from build123d import *

# Parameters (mm, degrees)
BOX_W              = 10
BOX_H              = 10
BOX_DEPTH          = 10
SKETCH_W           = 4.4
SKETCH_H           = 4.4
PAD_DEPTH          = 4
PAD_FACE4_W        = 10
PAD_FACE4_H        = 10
POCKET_DEPTH       = 2.5
POCKET_FACE5_W     = 10
POCKET_FACE5_H     = 10
POCKET001_DEPTH    = 2.5
SKETCH001_W        = 5
SKETCH001_H        = 10
PAD001_DEPTH       = 10
SKETCH002_W        = 4.4
SKETCH002_H        = 4.4
PAD002_DEPTH       = 4
PAD002_FACE22_W    = 4.4
PAD002_FACE22_H    = 4.4
POCKET002_DEPTH    = 5
POCKET002_FACE16_W = 5
POCKET002_FACE16_H = 10
POCKET003_DEPTH    = 7.5
POCKET003_FACE15_W = 5
POCKET003_FACE15_H = 10
POCKET004_DEPTH    = 2.5
POCKET005_DEPTH    = 9
POCKET005_FACE8_W  = 5
POCKET005_FACE8_H  = 1
PAD003_DEPTH       = 10
PAD003_FACE3_W     = 2.5
PAD003_FACE3_H     = 1
PAD004_DEPTH       = 15
PAD004_FACE7_W     = 5
PAD004_FACE7_H     = 1
PAD005_DEPTH       = 15
PAD005_FACE8_W     = 2.5
PAD005_FACE8_H     = 1
PAD006_DEPTH       = 15
PAD006_FACE23_W    = 10
PAD006_FACE23_H    = 1
PAD007_DEPTH       = 15
SKETCH003_W        = 4.4
SKETCH003_H        = 4.4
PAD008_DEPTH       = 4
PAD008_FACE15_W    = 2.5
PAD008_FACE15_H    = 1
POCKET006_DEPTH    = 2.5
POCKET006_FACE20_W = 5
POCKET006_FACE20_H = 1
POCKET007_DEPTH    = 2.5
POCKET007_FACE27_W = 2.5
POCKET007_FACE27_H = 1
POCKET008_DEPTH    = 2.5
POCKET008_FACE37_W = 10
POCKET008_FACE37_H = 1
POCKET009_DEPTH    = 2.5
POCKET009_FACE5_W  = 10
POCKET009_FACE5_H  = 1
PAD009_DEPTH       = 2.5
PAD009_FACE29_W    = 10
PAD009_FACE29_H    = 1
PAD010_DEPTH       = 2.5
POCKET010_DEPTH    = 5


with BuildPart() as part:
    # Box → Box (new body)
    with BuildSketch(Plane.XY):
        with Locations((5, 5)):
            Rectangle(BOX_W, BOX_H)
    extrude(amount=BOX_DEPTH)

    # Sketch (on Face6 of BaseFeature) → Pad (new body)
    with BuildSketch(Plane.XY.offset(10)):
        with Locations((5, 5)):
            Rectangle(SKETCH_W, SKETCH_H)
    extrude(amount=PAD_DEPTH)

    # Pad Face4 → Pocket (cut)
    with BuildSketch(Plane(origin=(5, 10, 5), x_dir=(1, 0, 0), z_dir=(0, 1, 0))):
        Rectangle(PAD_FACE4_W, PAD_FACE4_H)
    extrude(amount=-POCKET_DEPTH, mode=Mode.SUBTRACT)

    # Pocket Face5 → Pocket001 (cut)
    with BuildSketch(Plane(origin=(5, 0, 5), x_dir=(-1, 0, 0), z_dir=(0, -1, 0))):
        Rectangle(POCKET_FACE5_W, POCKET_FACE5_H)
    extrude(amount=-POCKET001_DEPTH, mode=Mode.SUBTRACT)

    # Sketch001 (on Face3 of Pocket001) → Pad001 (join)
    with BuildSketch(Plane(origin=(0, 7.5, 0), x_dir=(-1, 0, 0), z_dir=(0, 1, 0))):
        with Locations((-5, 5)):
            Rectangle(SKETCH001_W, SKETCH001_H)
    extrude(amount=PAD001_DEPTH)

    # Sketch002 (on Face6 of Pad001) → Pad002 (join)
    with BuildSketch(Plane.XY.offset(10)):
        with Locations((5, 12.5)):
            Rectangle(SKETCH002_W, SKETCH002_H)
    extrude(amount=PAD002_DEPTH)

    # Pad002 Face22 → Pocket002 (cut)
    with BuildSketch(Plane(origin=(5, 12.5, 14), x_dir=(0, 1, 0), z_dir=(0, 0, 1))):
        Rectangle(PAD002_FACE22_W, PAD002_FACE22_H)
    extrude(amount=-POCKET002_DEPTH, mode=Mode.SUBTRACT)

    # Pocket002 Face16 → Pocket003 (cut)
    with BuildSketch(Plane(origin=(5, 17.5, 5), x_dir=(1, 0, 0), z_dir=(0, 1, 0))):
        Rectangle(POCKET002_FACE16_W, POCKET002_FACE16_H)
    extrude(amount=-POCKET003_DEPTH, mode=Mode.SUBTRACT)

    # Pocket003 Face15 → Pocket004 (cut)
    with BuildSketch(Plane(origin=(5, 10, 5), x_dir=(1, 0, 0), z_dir=(0, 1, 0))):
        Rectangle(POCKET003_FACE15_W, POCKET003_FACE15_H)
    extrude(amount=-POCKET004_DEPTH, mode=Mode.SUBTRACT)

    # Pocket004 Face4 → Pocket005 (cut)
    with BuildSketch(Plane(origin=(5, 5, 0), x_dir=(0, -1, 0), z_dir=(0, 0, -1))):
        Polygon((2.5, 5), (-2.5, 5), (-2.5, 2.5), (-2.5, -2.5), (-2.5, -5), (2.5, -5), align=None)
    extrude(amount=-POCKET005_DEPTH, mode=Mode.SUBTRACT)

    # Pocket005 Face8 → Pad003 (add)
    with BuildSketch(Plane(origin=(10, 5, 9.5), x_dir=(0, -1, 0), z_dir=(1, 0, 0))):
        Rectangle(POCKET005_FACE8_W, POCKET005_FACE8_H)
    extrude(amount=PAD003_DEPTH)

    # Pad003 Face3 → Pad004 (add)
    with BuildSketch(Plane(origin=(1.25, 7.5, 9.5), x_dir=(1, 0, 0), z_dir=(0, 1, 0))):
        Rectangle(PAD003_FACE3_W, PAD003_FACE3_H)
    extrude(amount=PAD004_DEPTH)

    # Pad004 Face7 → Pad005 (add)
    with BuildSketch(Plane(origin=(5, 7.5, 9.5), x_dir=(1, 0, 0), z_dir=(0, 1, 0))):
        Rectangle(PAD004_FACE7_W, PAD004_FACE7_H)
    extrude(amount=PAD005_DEPTH)

    # Pad005 Face8 → Pad006 (add)
    with BuildSketch(Plane(origin=(8.75, 7.5, 9.5), x_dir=(1, 0, 0), z_dir=(0, 1, 0))):
        Rectangle(PAD005_FACE8_W, PAD005_FACE8_H)
    extrude(amount=PAD006_DEPTH)

    # Pad006 Face23 → Pad007 (add)
    with BuildSketch(Plane(origin=(15, 7.5, 9.5), x_dir=(1, 0, 0), z_dir=(0, 1, 0))):
        Rectangle(PAD006_FACE23_W, PAD006_FACE23_H)
    extrude(amount=PAD007_DEPTH)

    # Sketch003 (on Face9 of Pad007) → Pad008 (join)
    with BuildSketch(Plane.XY.offset(10)):
        with Locations((5, 15)):
            Rectangle(SKETCH003_W, SKETCH003_H)
        with Locations((15, 5)):
            Rectangle(SKETCH003_W, SKETCH003_H)
    extrude(amount=PAD008_DEPTH)

    # Pad008 Face15 → Pocket006 (cut)
    with BuildSketch(Plane(origin=(1.25, 22.5, 9.5), x_dir=(1, 0, 0), z_dir=(0, 1, 0))):
        Rectangle(PAD008_FACE15_W, PAD008_FACE15_H)
    extrude(amount=-POCKET006_DEPTH, mode=Mode.SUBTRACT)

    # Pocket006 Face20 → Pocket007 (cut)
    with BuildSketch(Plane(origin=(5, 22.5, 9.5), x_dir=(1, 0, 0), z_dir=(0, 1, 0))):
        Rectangle(POCKET006_FACE20_W, POCKET006_FACE20_H)
    extrude(amount=-POCKET007_DEPTH, mode=Mode.SUBTRACT)

    # Pocket007 Face27 → Pocket008 (cut)
    with BuildSketch(Plane(origin=(8.75, 22.5, 9.5), x_dir=(1, 0, 0), z_dir=(0, 1, 0))):
        Rectangle(POCKET007_FACE27_W, POCKET007_FACE27_H)
    extrude(amount=-POCKET008_DEPTH, mode=Mode.SUBTRACT)

    # Pocket008 Face37 → Pocket009 (cut)
    with BuildSketch(Plane(origin=(15, 22.5, 9.5), x_dir=(1, 0, 0), z_dir=(0, 1, 0))):
        Rectangle(POCKET008_FACE37_W, POCKET008_FACE37_H)
    extrude(amount=-POCKET009_DEPTH, mode=Mode.SUBTRACT)

    # Pocket009 Face5 → Pad009 (add)
    with BuildSketch(Plane(origin=(5, 2.5, 9.5), x_dir=(-1, 0, 0), z_dir=(0, -1, 0))):
        Rectangle(POCKET009_FACE5_W, POCKET009_FACE5_H)
    extrude(amount=PAD009_DEPTH)

    # Pad009 Face29 → Pad010 (add)
    with BuildSketch(Plane(origin=(15, 2.5, 9.5), x_dir=(-1, 0, 0), z_dir=(0, -1, 0))):
        Rectangle(PAD009_FACE29_W, PAD009_FACE29_H)
    extrude(amount=PAD010_DEPTH)

    # Sketch004 (on Face4 of Pad010) → Pocket010 (cut)
    with BuildSketch(Plane(origin=(0, 0, 9), x_dir=(1, 0, 0), z_dir=(0, 0, -1))):
        with BuildLine():
            ThreePointArc((-0.886172, -19.999824), (13.825198, -14.457891), (19.99786, 0.000176))
            Line((19.99786, 0.000176), (29.314018, -0.170935))
            Line((29.314018, -0.170935), (32.97797, -26.044666))
            Line((32.97797, -26.044666), (-1.074295, -29.619213))
            Line((-1.074295, -29.619213), (-0.886172, -19.999824))
        make_face()
    extrude(amount=-POCKET010_DEPTH, mode=Mode.SUBTRACT)


solid = part.part
Model file for the job. Use its own axes, mm. A direction names the side the tool comes from. Round coordinates to 2 decimals unless told otherwise and drop trailing zeros. Loops run counter-clockwise (first coordinate to the right, second up) from the corner with the lowest first, then second, coordinate; pieces in that order, holes last.
1. Drop flat-ended pins along their axis: P1, Ø1.2, axis at y = 14.5, z = 12.5, coming from the +X side; P2, Ø2, axis at y = 15, z = 13, coming from the -X side; P3, Ø1.5, axis at x = 16.5, z = 13, coming from the -Y side. Give the stop position or say it passes through.
Check values:
P1: stops at x = 7.2
P2: stops at x = 2.8
P3: stops at y = 2.8
2. Band-saw the part on B-B, the plane y = 16. List the corners of the cut face in (x, z), and give its area (3 significant figures).
Check values:
outline: (0, 9) - (12.01, 9) - (12.01, 10) - (7.2, 10) - (7.2, 14) - (2.8, 14) - (2.8, 10) - (0, 10) - close
area: 29.6 mm2
3. Tool access for faces 1 (the flat face through (7.2, 15, 12)), 2 (the flat face through (12.8, 5, 12)), 3 (the flat face through (5, 17.2, 12)), 4 (the flat face through (15, 2.8, 12)), 5 (the flat face through (2.8, 15, 12)): list every direction of +Z, -Z, +X, -X, +Y, -Y with a clear straight run to the whole face (end or side of a thin tool).
Check values:
face 1: +Z, +X, +Y, -Y
face 2: +Z, +Y, -Y
face 3: +Z, +X, -X, +Y
face 4: +Z, +X, -X, -Y
face 5: +Z, -X, +Y, -Y
4. Band-saw the part on C-C, the plane x = 3.75. List the corners of the cut face in (y, z), and give its area (3 significant figures).
Check values:
outline: (0, 9) - (19.66, 9) - (19.66, 10) - (17.2, 10) - (17.2, 14) - (12.8, 14) - (12.8, 10) - (7.2, 10) - (7.2, 14) - (2.8, 14) - (2.8, 10) - (0, 10) - close
area: 54.9 mm2
5. Band-saw the part on A-A, the plane z = 12.2. List the corners of the cut face in (x, y).
Check values:
outline: (2.8, 2.8) - (7.2, 2.8) - (7.2, 7.2) - (2.8, 7.2) - close; (2.8, 12.8) - (7.2, 12.8) - (7.2, 17.2) - (2.8, 17.2) - close; (12.8, 2.8) - (17.2, 2.8) - (17.2, 7.2) - (12.8, 7.2) - close
6. Wall check: probe 1 along Y at (x, z) = (5.75, 11.8); probe 2 along Z at (x, y) = (4.75, 17.5). Give the ranges that are in metal, low to high.
Check values:
probe 1: y = 2.8 to 7.2, 12.8 to 17.2
probe 2: z = 9 to 10
7. Band-saw the part on D-D, the plane z = 9.55. List the corners of the cut face in (x, y), and give its area (3 significant figures).
Check values:
outline: (0, 0) - (20, 0) arc R20.02 ccw to (0.84, 20) - (0, 20) - close
area: 314 mm2
